Part print with two shaded views. Sizes in mm from the minimum x, y, z corner. A direction names the side the tool comes from. Give positions to 0.01 mm unless a question says otherwise; leave off trailing zeros. Write each loop counter-clockwise with the first axis right and the second up, starting at its lowest first coordinate (ties: lowest second). Pieces come first, ordered by that corner, then holes. Notation, with made-up numbers: (88, -37.5) -> (138, -37.5) arc R18 ccw to (138, -2.5) -> close; hole circle Ø10 at (23, 15.5). An arc over 180 degrees is marked (long way). Use one line per item in the form item = value. Start each with the question number.
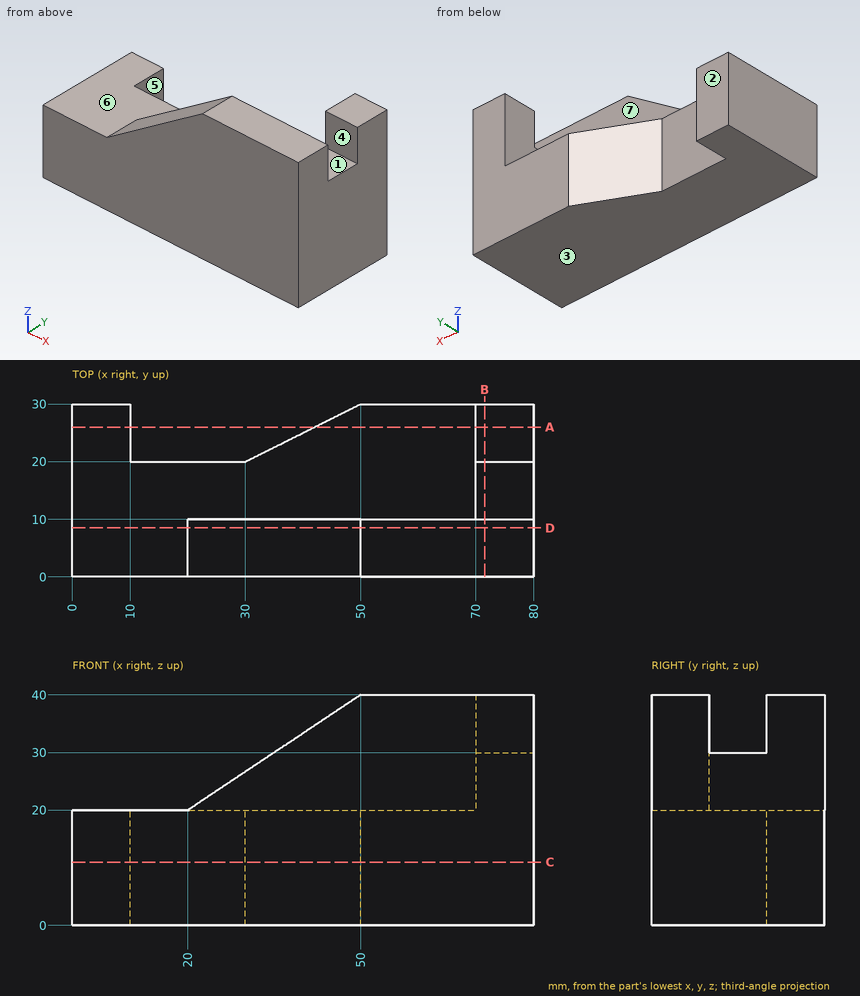
1) Cut at D-D (y = 8.5). Give the cut face in (x, z).
2) Cut at A-A (y = 26). Give the cut face in (x, z), and give its area (3 significant figures).
3) Cut at B-B (x = 71.5). Give the cut face in (y, z), and give its area (3 significant figures).
4) Cut at C-C (z = 11). Give the cut face in (x, y).
5) 3-axis set-ups, long thin cutter, end or side, ignore diameter. For the marked faces 5, 6 and 7: which of +Z, -Z, +X, -X, +Y, -Y reach the whole face in a straight line?
6) Two-plate mould, pull along Y, no slides. Class the marked faces 1, 2, 3 and 4: released by +Y, released by -Y, zero draft, split by the parting line, or undercut.
7) Pin check, flat tips, straight feed: pin 1 (6 mm diameter, centred on y = 22.5, z = 31.5, fed in from -X); pin 2 (6 mm diameter, centred on x = 55.5, z = 30, fed in from +Y); pin 3 (1 mm diameter, centred on x = 58, y = 19.5, fed in from -Z); pin 4 (10 mm diameter, centred on x = 22, z = 6.5, fed in from +Y). Stop position of each tip, or through.
8) Wall check: line 1 along Z through (x, y) = (65, 15); line 2 along X through (y, z) = (27.5, 25); line 3 along X through (y, z) = (24.5, 18). Give the ranges that are in metal, low to high. Write a range as from..to.
Final values:
q1.outline = (0, 0) -> (80, 0) -> (80, 40) -> (50, 40) -> (20, 20) -> (0, 20) -> close
q2.outline = (0, 0) -> (10, 0) -> (10, 20) -> (0, 20) -> close; (42, 0) -> (80, 0) -> (80, 40) -> (70, 40) -> (70, 20) -> (42, 20) -> close
q2.area = 1,160 mm^2
q3.outline = (0, 0) -> (30, 0) -> (30, 40) -> (20, 40) -> (20, 30) -> (10, 30) -> (10, 40) -> (0, 40) -> close
q3.area = 1,100 mm^2
q4.outline = (0, 0) -> (80, 0) -> (80, 30) -> (50, 30) -> (30, 20) -> (10, 20) -> (10, 30) -> (0, 30) -> close
q5.face_5 = +Z, -Z, +Y
q5.face_6 = +Z, -X, +Y
q5.face_7 = +Z, -X
q6.face_1 = undercut
q6.face_2 = released by +Y
q6.face_3 = zero draft
q6.face_4 = undercut
q7.pin_1 = 70
q7.pin_2 = 10
q7.pin_3 = 0
q7.pin_4 = 20
q8.line_1 = 0..20
q8.line_2 = 70..80
q8.line_3 = 0..10, 39..80
